```python
from build123d import *

# Parameters (mm, degrees)
SKETCH_1_R          = 40
EXTRUDE_1_DEPTH     = 12
SKETCH_8_R          = 45
EXTRUDE_3_DEPTH     = 2
SKETCH_2_R          = 7.5
CUT_EXTRUDE_1_DEPTH = 66.161338231
HOLE_WIZARD_M32_D   = 3.4
CUT_EXTRUDE_2_DEPTH = 66.161338231
M3X0_51_D           = 2.5
SKETCH_18_R         = 17.5
CUT_EXTRUDE_4_DEPTH = 1
FILLET_1_R          = 2


with BuildPart() as part:
    # Эскиз1 → Бобышка-Вытянуть1 (new body)
    with BuildSketch(Plane.XY):
        Circle(SKETCH_1_R)
    extrude(amount=EXTRUDE_1_DEPTH)

    # Эскиз8 → Бобышка-Вытянуть3 (add)
    with BuildSketch(Plane.XY.offset(12)):
        Circle(SKETCH_8_R)
    extrude(amount=EXTRUDE_3_DEPTH)

    # Эскиз2 → Вырез-Вытянуть1 (cut, through all)
    with BuildSketch(Plane(origin=(0, 0, 14), x_dir=(-1, 0, 0), z_dir=(0, 0, -1))):
        Circle(SKETCH_2_R)
    extrude(amount=CUT_EXTRUDE_1_DEPTH, mode=Mode.SUBTRACT)

    # Отверстие с зазором M32 (through all)
    with Locations(Plane.XY.offset(14)):
        with Locations((6.25, 10.825317547), (-12.5, 0), (6.25, -10.825317547)):
            Hole(HOLE_WIZARD_M32_D / 2)

    # Эскиз10 → Вырез-Вытянуть2 (cut, through all)
    with BuildSketch(Plane(origin=(0, 0, 0), x_dir=(-1, 0, 0), z_dir=(0, 0, -1))):
        with BuildLine():
            ThreePointArc((32.475952642, -18.75), (28.632685902, -4.40673326), (14.289419162, -8.25))
            ThreePointArc((14.289419162, -8.25), (8.25, -14.289419162), (0, -16.5))
            ThreePointArc((0, -16.5), (-10.5, -27), (0, -37.5))
            ThreePointArc((0, -37.5), (18.75, -32.475952642), (32.475952642, -18.75))
        make_face()
        with BuildLine():
            ThreePointArc((32.475952642, 18.75), (18.75, 32.475952642), (0, 37.5))
            ThreePointArc((0, 37.5), (-10.5, 27), (0, 16.5))
            ThreePointArc((0, 16.5), (8.25, 14.289419162), (14.289419162, 8.25))
            ThreePointArc((14.289419162, 8.25), (28.632685902, 4.40673326), (32.475952642, 18.75))
        make_face()
        with BuildLine():
            ThreePointArc((-32.475952642, -18.75), (-18.132685902, -22.59326674), (-14.289419162, -8.25))
            ThreePointArc((-14.289419162, -8.25), (-16.5, 0), (-14.289419162, 8.25))
            ThreePointArc((-14.289419162, 8.25), (-18.132685902, 22.59326674), (-32.475952642, 18.75))
            ThreePointArc((-32.475952642, 18.75), (-37.5, 0), (-32.475952642, -18.75))
        make_face()
    extrude(amount=-CUT_EXTRUDE_2_DEPTH, mode=Mode.SUBTRACT)

    # Отверстие обработанное метчиком M3x0.51 (through all)
    with Locations(Plane(origin=(0, 0, 0), x_dir=(-1, 0, 0), z_dir=(0, 0, -1))):
        with Locations((-17.5, 30.310889132), (35, 0), (-17.5, -30.310889132)):
            Hole(M3X0_51_D / 2)

    # Эскиз18 → Вырез-Вытянуть4 (cut)
    with BuildSketch(Plane(origin=(0, 0, 0), x_dir=(-1, 0, 0), z_dir=(0, 0, -1))):
        Circle(SKETCH_18_R)
    extrude(amount=-CUT_EXTRUDE_4_DEPTH, mode=Mode.SUBTRACT)

    # Скругление1
    fillet_1_edges = [part.edges().sort_by_distance(p)[0] for p in [
        (3.581311038, 17.12962963, 0.5),
        (-16.625349936, 5.463308477, 0.5),
        (-16.625349936, -5.463308477, 0.5),
        (3.581311038, -17.12962963, 0.5),
        (13.044038898, -11.666321153, 0.5),
        (13.044038898, 11.666321153, 0.5),
    ]]
    fillet(fillet_1_edges, radius=FILLET_1_R)


solid = part.part
```
Could you check a few things on this model? Use its own coordinates, in mm. A direction names the side the tool comes from. Give positions to 0.01 mm unless a question says otherwise; leave off trailing zeros. Order: outer loops, then holes, each group sorted by start corner. A loop starts at its lowest first (then second) coordinate and runs counter-clockwise, first axis right, second up.
Q1. For faces 4 (the cylindrical face through (-8.67, -39.05, 5.92)), 5 (the flat face through (9, 1, 14)), 6 (the cylindrical face through (37.5, 0.3, 6.9)), which set-ups out of +Z, -Z, +X, -X, +Y, -Y let a thin tool reach every point of the face, with its end or its side?
Q2. Suppose I cut it at C-C, the plane x = 27.5. Write out the boundary of the cut face in (y, z), and give its area (3 significant figures).
Q3. Suppose I cut it at B-B, the plane y = -21. Write out the boundary of the cut face in (x, z).
Q4. Suppose I cut it at D-D, the plane z = 2.5. Count the separate pieces of the cut face and the enclosed holes in it, and give its area (3 significant figures).
Q5. I'm going to push flat-ended pins straight in: P1, Ø4, axis at x = 6.25, y = 10.83, coming from the -Z side; P2, Ø6, axis at x = -7.5, z = 11.5, coming from the +Y side; P3, Ø1.5, axis at x = 31.5, z = 5.5, coming from the -Y side. Where does each tip first touch, or does it pass through?
Q6. Suppose I cut it at A-A, the plane y = 0. Write out the boundary of the cut face in (x, z).
Q7. If I drill on line 1 along Y through (x, z) = (-17.5, 9.5); line 2 along X through (y, z) = (-22, 13); line 3 along X through (y, z) = (5.5, 9.25), over which ranges is the centre line in solid material (lowest first)?
Q8. We'd pull the mould along X, two halves only. Please class faces 1 (the cylindrical face through (20.765, -39.923, 12.986)), 2 (the flat face through (-18, 0, 0)), 3 (the cylindrical face through (7.493, 0.33, 7.591)): +X half, -X half, draft (parallel to the pull), parting line (faces both ways), or undercut.
Solution:
1. face 4: -Z
1. face 5: +Z, +X, -X, +Y, -Y
1. face 6: +Z, -Z
2. outline: (-35.62, 12) - (-29.05, 12) - (-29.05, 0) - (-23.16, 0) - (-23.16, 14) - (-35.62, 14) - close; (23.16, 0) - (29.05, 0) - (29.05, 12) - (35.62, 12) - (35.62, 14) - (23.16, 14) - close
2. area: 191 mm2
3. outline: (-39.8, 12) - (-34.04, 12) - (-34.04, 0) - (-31.07, 0) - (-31.07, 14) - (-39.8, 14) - close; (8.62, 0) - (16.03, 0) - (16.03, 14) - (8.62, 14) - close; (30.73, 0) - (34.04, 0) - (34.04, 12) - (39.8, 12) - (39.8, 14) - (30.73, 14) - close
4. separate pieces: 1
4. enclosed holes: 10
4. area: 1,990 mm2
5. P1: stops at z = 1
5. P2: stops at y = 44.77
5. P3: stops at y = -25.58
6. outline: (-45, 12) - (-40, 12) - (-40, 0) - (-36.25, 0) - (-36.25, 14) - (-45, 14) - close; (-33.75, 0) - (-17.5, 0) - (-17.5, 1) - (-14.2, 1) - (-14.2, 14) - (-33.75, 14) - close; (-10.8, 1) - (-7.5, 1) - (-7.5, 14) - (-10.8, 14) - close; (7.5, 1) - (16.5, 1) - (16.5, 14) - (7.5, 14) - close; (37.5, 0) - (40, 0) - (40, 12) - (45, 12) - (45, 14) - (37.5, 14) - close
7. line 1: y = -35.97 to -33.17, -4.8 to 4.8, 33.17 to 35.97
7. line 2: x = -39.26 to -30.37, 9.23 to 17.22, 29.55 to 39.26
7. line 3: x = -39.62 to -30.18, -16.58 to -5.1, 5.1 to 15.56, 37.09 to 39.62
8. face 1: parting line
8. face 2: draft
8. face 3: undercut
